Geometry: see drawing. Coordinates: mm, zero at the bounding-box minimum. A direction names the side the tool comes from. Give positions to 0.01 mm unless a question says otherwise; leave off trailing zeros. Order: outer loops, then holes, each group sorted by start corner. A loop starts at its lowest first (then second) coordinate and runs counter-clockwise, first axis right, second up. Notation, with made-up numbers: (23, 7.25) - (70, 7.25) arc R32 ccw to (70, 41.25) - close; hole circle Ø9 at (0, -34). An arc over 180 degrees is marked (long way). Put each result on its own line as item: value. Start each with the question number.
1. Section C-C on z = 46. Return the cut outline in (x, y) (1 decimal).
2. Section B-B on y = 48.5. Return the cut outline in (x, z).
3. Section A-A on x = 76. Return the cut outline in (y, z), plus the area to 3 significant figures.
4. Section D-D on x = 127.5. Return the cut outline in (y, z).
5. First-contact query: P1, Ø1, axis at y = 17.5, z = 33, coming from the -X side (1 decimal); P2, Ø4, axis at x = 46.5, y = 44.5, coming from the +Z side (1 decimal); P3, Ø4, axis at x = 71, z = 8.5, coming from the -Y side. Flat tips, straight axial feed; report the tip coordinate or a pass-through.
6. Ray query, line 1 along Z through (x, y) = (68, 12); line 2 along Y through (x, z) = (60.5, 35); line 3 along X through (y, z) = (42.5, 35). Return the intervals inside material, ascending. Write a range as from..to.
7. Set-up query: the marked faces 1 and 2. Return all of +Z, -Z, +X, -X, +Y, -Y with unobstructed straight access to the full face (end or side cutting, diameter ignored); none if empty.
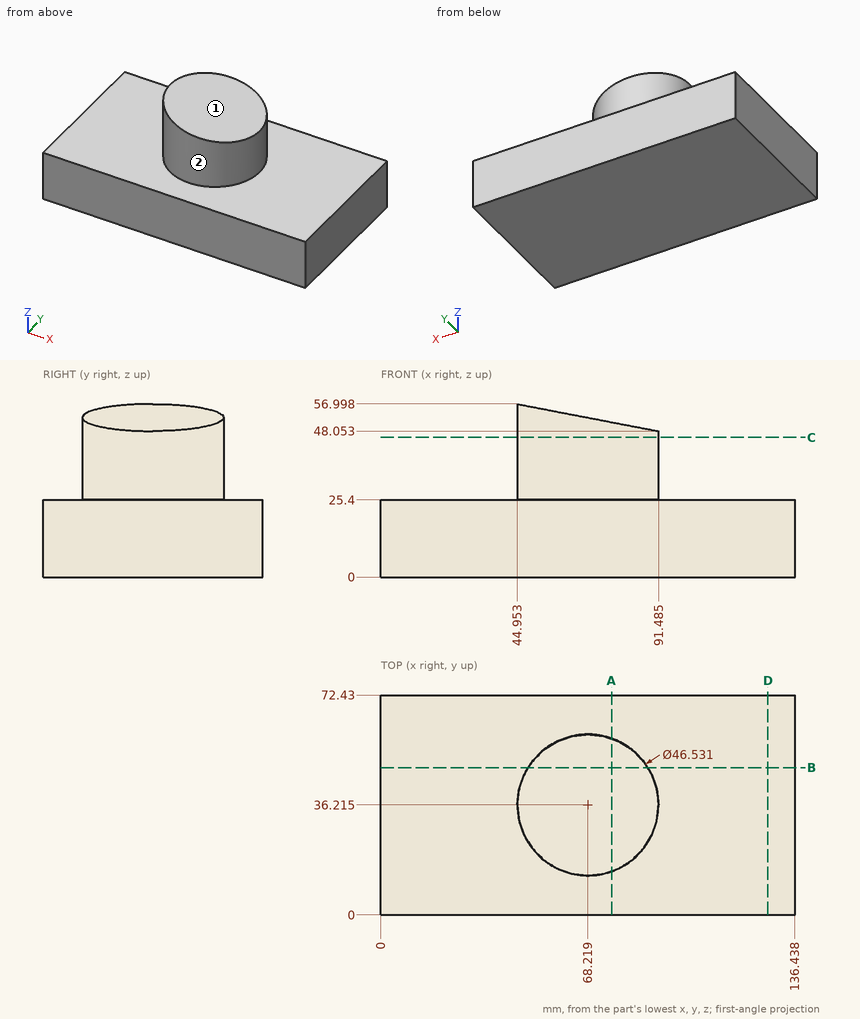
Resolved:
1. outline: circle Ø46.5 at (68.2, 36.2)
2. outline: (0, 0) - (136.44, 0) - (136.44, 25.4) - (87.98, 25.4) - (87.98, 48.73) - (48.46, 56.32) - (48.46, 25.4) - (0, 25.4) - close
3. outline: (0, 0) - (72.43, 0) - (72.43, 25.4) - (58.14, 25.4) - (58.14, 51.03) - (14.29, 51.03) - (14.29, 25.4) - (0, 25.4) - close
3. area: 2,960 mm^2
4. outline: (0, 0) - (72.43, 0) - (72.43, 25.4) - (0, 25.4) - close
5. P1: x = 53.7
5. P2: z = 56.8
5. P3: y = 0
6. line 1: 0..25.4
6. line 2: 14.27..58.16
6. line 3: 45.82..90.62
7. face 1: +Z, +X, +Y, -Y
7. face 2: +Z
